CAD build for the part. Positions are in the model's coordinates, mm. Coordinates: 2 decimals unless noted, no trailing zeros. Write each loop counter-clockwise with the first axis right and the second up, starting at its lowest first coordinate (ties: lowest second). Pieces come first, ordered by that corner, then holes. Notation, with made-up numbers: (12, 22) - (60, 22) arc R29 ccw to (60, 61) - close; hole circle Ø3 at (-29, 54.5). An arc over 180 degrees is marked (long way). One line per question, with ' | ' between items. Start each with the question number.
1. Band-saw the part on B-B, the plane y = 0.75. Write the cut outline in (x, z), then the cut area to 3 significant figures.
2. Two-plate mould, pull along X, no slides. Class faces 1 (the flat face through (-10, 7.5, -29)), 2 (the cylindrical face through (-4.39, 3.7, -27.73)), 3 (the flat face through (22.5, 4, -34)): +X half, -X half, draft (parallel to the pull), parting line (faces both ways), or undercut.
3. Band-saw the part on C-C, the plane z = -47.5. Write the cut outline in (x, y).
4. Band-saw the part on A-A, the plane x = 0. Write the cut outline in (y, z).
5. Probe line 1 (X direction, y = 5.5, z = -47.5); line 2 (Z direction, x = 0, y = 2); line 3 (X direction, y = 5.75, z = -51.5). List the from-to ranges inside material, lowest first.
from build123d import *

# Parameters (mm, degrees)
SKETCH1_W           = 45
SKETCH1_H           = 73
SKETCH1_R           = 20.25
BOSS_EXTRUDE1_DEPTH = 7.5
CHAMFER1_SIZE       = 4


with BuildPart() as part:
    # Sketch1 → Boss-Extrude1 (new body)
    with BuildSketch(Plane(origin=(0, 0, 0), x_dir=(1, 0, 0), z_dir=(0, 1, 0))):
        with Locations((0, 36.5)):
            Rectangle(SKETCH1_W, SKETCH1_H)
        with Locations((0, 47.5)):
            Circle(SKETCH1_R, mode=Mode.SUBTRACT)
    extrude(amount=BOSS_EXTRUDE1_DEPTH)

    # Chamfer1
    chamfer1_edges = [part.edges().sort_by_distance(p)[0] for p in [
        (-22.5, 3.75, -73),
        (22.5, 3.75, -73),
    ]]
    chamfer(chamfer1_edges, length=CHAMFER1_SIZE)


solid = part.part
Filled in:
1) outline: (-22.5, -69) - (-18.5, -73) - (18.5, -73) - (22.5, -69) - (22.5, 0) - (-22.5, 0) - close; hole circle Ø40.5 at (0, -47.5) | area: 1,980 mm²
2) face 1: draft | face 2: undercut | face 3: +X half
3) outline: (-22.5, 0) - (-20.25, 0) - (-20.25, 7.5) - (-22.5, 7.5) - close; (20.25, 0) - (22.5, 0) - (22.5, 7.5) - (20.25, 7.5) - close
4) outline: (0, -73) - (7.5, -73) - (7.5, -67.75) - (0, -67.75) - close; (0, -27.25) - (7.5, -27.25) - (7.5, 0) - (0, 0) - close
5) line 1: x = -22.5 to -20.25, 20.25 to 22.5 | line 2: z = -73 to -67.75, -27.25 to 0 | line 3: x = -22.5 to -19.85, 19.85 to 22.5
